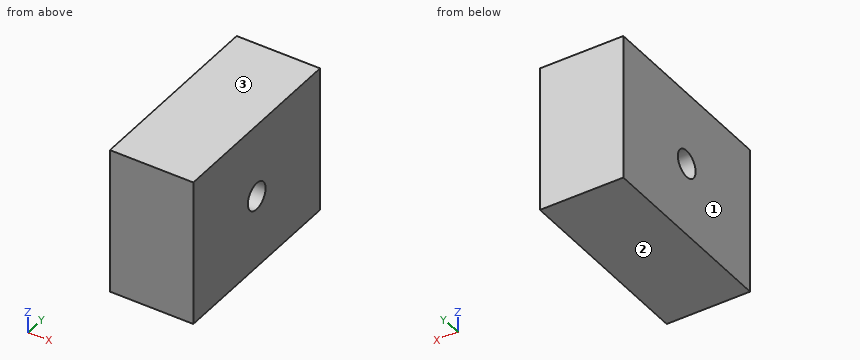
```python
from build123d import *

# Parameters (mm, degrees)
F0_W     = 10.8
F0_H     = 25
F1_DEPTH = 19
F3_D     = 3.5
F3_DEPTH = 20


with BuildPart() as f1:
    # F0 (on Top) → F1 (new body)
    with BuildSketch(Plane.XY):
        with Locations((-1.690517, -19.583154)):
            Rectangle(F0_W, F0_H)
    extrude(amount=F1_DEPTH)

    # F3
    with Locations(Plane.YZ.offset(3.709483)):
        with Locations((-19.583154, 9.5)):
            Hole(F3_D / 2, depth=F3_DEPTH)


solid = f1.part
```
The listing builds one solid part. Answer for the finished solid, in the listing's coordinates (mm). Face numbers are marked on the shaded views. Round coordinates to 2 decimals unless told otherwise and drop trailing zeros. Write each loop counter-clockwise with the first axis right and the second up, starting at its lowest first coordinate (ties: lowest second). Pieces come first, ordered by that corner, then holes. Notation, with made-up numbers: (72, 47.25) -> (120, 47.25) arc R17 cw to (120, 67.25) -> close; hole circle Ø8 at (54, 73). An arc over 180 degrees is marked (long way). Use CSV: the item, a comma, the result in double quotes. Start each with the question number.
(1) Section B-B on y = -19.5 is taken. Give the vertices of the cut face in (x, z), then the cut area to 3 significant figures.
(2) Section A-A on z = 9.5 is taken. Give the vertices of the cut face in (x, y).
(3) This flat-tipped pin is pushed along its axis until it touches: pin 1 (2 mm diameter, centred on y = -19.58, z = 9.5, fed in from -X). Where does it stop, or does it pass through?
(4) Consider L1, parallel to Z at x = -1.5, y = -19.5; L2, parallel to Z at x = -4, y = -20.25. Determine where each line is inside the solid, lowest interval first. Write a range as from..to.
(5) Section C-C on x = -0.25 is taken. Give the vertices of the cut face in (y, z).
(6) The mould has two halves that part along Z. Classify the marked faces 1, 2 and 3: released by +Z, released by -Z, zero draft, split by the parting line, or undercut.
A:
1,outline,"(-7.09, 0) -> (3.71, 0) -> (3.71, 7.75) -> (-7.09, 7.75) -> close; (-7.09, 11.25) -> (3.71, 11.25) -> (3.71, 19) -> (-7.09, 19) -> close"
1,area,"167 mm²"
2,outline,"(-7.09, -32.08) -> (3.71, -32.08) -> (3.71, -21.33) -> (-7.09, -21.33) -> close; (-7.09, -17.83) -> (3.71, -17.83) -> (3.71, -7.08) -> (-7.09, -7.08) -> close"
3,pin 1,"passes through"
4,L1,"z = 0..7.75, 11.25..19"
4,L2,"z = 0..7.88, 11.12..19"
5,outline,"(-32.08, 0) -> (-7.08, 0) -> (-7.08, 19) -> (-32.08, 19) -> close; hole circle Ø3.5 at (-19.58, 9.5)"
6,face 1,"zero draft"
6,face 2,"released by -Z"
6,face 3,"released by +Z"
